For this review, take the finished solid that the model builds, in its own axes (mm). Face numbers are marked on the shaded views. A direction names the side the tool comes from. Round coordinates to 2 decimals unless told otherwise and drop trailing zeros. Write each loop counter-clockwise with the first axis right and the second up, starting at its lowest first coordinate (ties: lowest second). Pieces come first, ordered by that corner, then holes. Notation, with made-up numbers: (17.5, -15.75) - (73.5, -15.75) arc R27 ccw to (73.5, 4.25) - close; hole circle Ø1 at (55, 39). An arc over 180 degrees is marked (long way). One line per item, written item: value. Start each with the question number.
Q1. Mouldability with a two-part tool opening along Y and no side actions: class the marked faces 1, 2 and 3 as +Y half, -Y half, draft (parallel to the pull), parting line (faces both ways), or undercut.
Q2. For probe 1 along Z at (x, y) = (29.5, 12.5); probe 2 along Y at (x, z) = (0, 8.75); probe 3 along Y at (x, z) = (0, 0.85), list the stretches that pass through material, from the lowest coordinate up.
Q3. Add section D-D on y = -16.5. Write out the cut boundary in (x, z), and give its area (3 significant figures).
Q4. Add section A-A on x = 0. Write out the cut boundary in (y, z).
Q5. Clearance check with flat-ended pins moving along their axes: pin 1 Ø19 at (x, y) = (0, 0) entering from -Z; pin 2 Ø1.5 at (x, z) = (-19.5, 3.5) entering from -Y; pin 3 Ø4 at (x, z) = (-13.5, 4.5) entering from -Y. State where each tip first meets the part, or that it passes through.
Q6. Tool access review of the marked faces 4 and 5: name each direction out of +Z, -Z, +X, -X, +Y, -Y from which nothing blocks a thin tool from reaching the whole face with its end or side.
Q7. Add section C-C on z = 4.5. Write out the cut boundary in (x, y).
```python
from build123d import *

# Parameters (mm, degrees)
SKETCH_1_R          = 30.47
EXTRUDE_1_DEPTH     = 13
SKETCH_2_R          = 33.47
EXTRUDE_2_DEPTH     = 1.5
EXTRUDE_START       = 1.5
SKETCH_3_R          = 33.47
EXTRUDE_3_DEPTH     = 1.5
SKETCH_4_R          = 6
CUT_EXTRUDE_1_DEPTH = 50.964805614
SKETCH_5_R          = 10
CUT_EXTRUDE_2_DEPTH = 5


with BuildPart() as part:
    # 草图1 → 凸台-拉伸1 (new body)
    with BuildSketch(Plane.XY):
        with Locations(Location((0, 0, 0), (0, 0, 180))):
            Circle(SKETCH_1_R)
    extrude(amount=EXTRUDE_1_DEPTH)

    # 草图2 → 凸台-拉伸2 (add)
    with BuildSketch(Plane.XY.offset(13)):
        Circle(SKETCH_2_R)
    extrude(amount=EXTRUDE_2_DEPTH)

    # 草图3 → 凸台-拉伸3 (add)
    with BuildSketch(Plane(origin=(0, 0, 0), x_dir=(-1, 0, 0), z_dir=(0, 0, -1)).offset(EXTRUDE_START)):
        with Locations(Location((0, 0, 0), (0, 0, 180))):
            Circle(SKETCH_3_R)
    extrude(amount=-EXTRUDE_3_DEPTH)

    # 草图4 → 切除-拉伸1 (cut, through all)
    with BuildSketch(Plane(origin=(0, 0, -1.5), x_dir=(-1, 0, 0), z_dir=(0, 0, -1))):
        Circle(SKETCH_4_R)
    extrude(amount=-CUT_EXTRUDE_1_DEPTH, mode=Mode.SUBTRACT)

    # 草图5 → 切除-拉伸2 (cut)
    with BuildSketch(Plane(origin=(0, 0, -1.5), x_dir=(-1, 0, 0), z_dir=(0, 0, -1))):
        Circle(SKETCH_5_R)
    extrude(amount=-CUT_EXTRUDE_2_DEPTH, mode=Mode.SUBTRACT)


solid = part.part
```
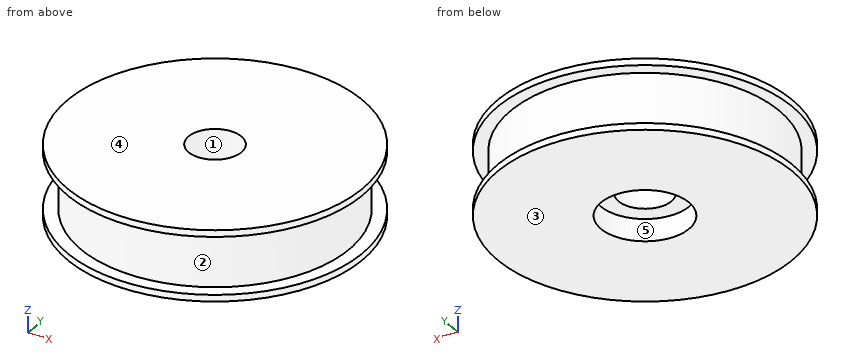
Result set:
1. face 1: undercut
1. face 2: parting line
1. face 3: draft
2. probe 1: z = -1.5 to 0, 13 to 14.5
2. probe 2: y = -30.47 to -6, 6 to 30.47
2. probe 3: y = -30.47 to -10, 10 to 30.47
3. outline: (-29.12, -1.5) - (29.12, -1.5) - (29.12, 0) - (25.62, 0) - (25.62, 13) - (29.12, 13) - (29.12, 14.5) - (-29.12, 14.5) - (-29.12, 13) - (-25.62, 13) - (-25.62, 0) - (-29.12, 0) - close
3. area: 841 mm^2
4. outline: (-33.47, -1.5) - (-10, -1.5) - (-10, 3.5) - (-6, 3.5) - (-6, 14.5) - (-33.47, 14.5) - (-33.47, 13) - (-30.47, 13) - (-30.47, 0) - (-33.47, 0) - close; (6, 3.5) - (10, 3.5) - (10, -1.5) - (33.47, -1.5) - (33.47, 0) - (30.47, 0) - (30.47, 13) - (33.47, 13) - (33.47, 14.5) - (6, 14.5) - close
5. pin 1: stops at z = 3.5
5. pin 2: stops at y = -24.02
5. pin 3: stops at y = -28.22
6. face 4: +Z, +X, -X, +Y, -Y
6. face 5: -Z
7. outline: circle Ø60.94 at (0, 0); hole circle Ø12 at (0, 0)
